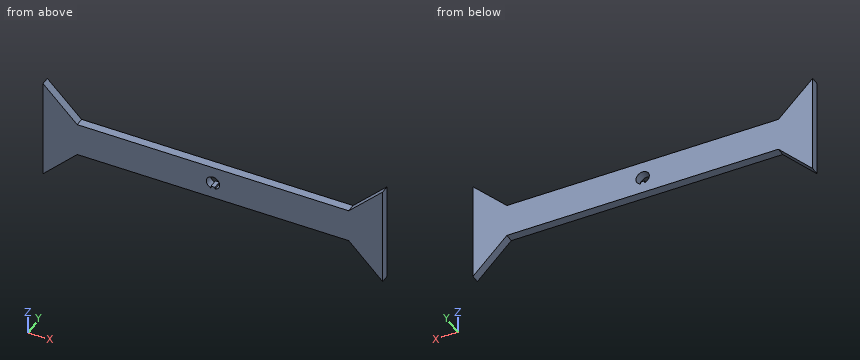
```python
from build123d import *

# Parameters (mm, degrees)
BOSS_EXTRUDE2_DEPTH = 6.35


with BuildPart() as part:
    # Sketch1 → Boss-Extrude2 (new body)
    with BuildSketch(Plane(origin=(0, 0, 0), x_dir=(1, 0, 0), z_dir=(0, 1, 0))):
        Polygon((0, 51.029291752), (0, -25.629291752), (25.629291752, 0), (228.829291752, 0), (254.229291752, -25.094710057), (254.229291752, 51.105289943), (228.829291752, 25.4), (25.629291752, 25.4), align=None)
        with BuildLine():
            Line((125.729291752, 17.77498595), (125.729291752, 16.205289943))
            Line((125.729291752, 16.205289943), (128.729291752, 16.205289943))
            Line((128.729291752, 16.205289943), (128.729291752, 17.77498595))
            ThreePointArc((128.729291752, 17.77498595), (127.229291752, 8.005289943), (125.729291752, 17.77498595))
        make_face(mode=Mode.SUBTRACT)
    extrude(amount=BOSS_EXTRUDE2_DEPTH)


solid = part.part
```
Read the model definition and answer for the solid it produces. Units are mm, in the model's axes. Give positions to 0.01 mm unless a question says otherwise; leave off trailing zeros. Loops run counter-clockwise (first coordinate to the right, second up) from the corner with the lowest first, then second, coordinate; pieces in that order, holes last.
Item 1: The part is cut by section D-D (x = 210). Write down the section's boundary in (y, z), and give its area (3 significant figures).
Item 2: The part is cut by section A-A (y = 2). Write down the section's boundary in (x, z), and give its area (3 significant figures).
Item 3: The part is cut by section C-C (z = 9). Write down the section's boundary in (x, y).
Item 4: Each of these flat-tipped pins is pushed along its axis until it touches: pin 1 Ø1.5 at (x, y) = (211, 1) entering from -Z; pin 2 Ø3.5 at (x, y) = (127, 3) entering from +Z. Where does it stop, or does it pass through?
Item 5: The part is cut by section B-B (z = -12). Write down the section's boundary in (x, y), and give its area (3 significant figures).
Item 6: Find the intervals of material crossed by line 1 along Z through (x, y) = (120, 1.75); line 2 along Z through (x, y) = (131.5, 3.25); line 3 along X through (y, z) = (3, -35), in increasing order.
Taken from the geometry:
1. outline: (0, -25.4) - (6.35, -25.4) - (6.35, 0) - (0, 0) - close
1. area: 161 mm2
2. outline: (0, -51.03) - (25.63, -25.4) - (228.83, -25.4) - (254.23, -51.11) - (254.23, 25.09) - (228.83, 0) - (25.63, 0) - (0, 25.63) - close; hole (125.73, -17.77) - (125.73, -16.21) - (128.73, -16.21) - (128.73, -17.77) arc R5 ccw (long way) to start
2. area: 7,690 mm2
3. outline: (0, 0) - (16.63, 0) - (16.63, 6.35) - (0, 6.35) - close; (237.94, 0) - (254.23, 0) - (254.23, 6.35) - (237.94, 6.35) - close
4. pin 1: stops at z = -25.4
4. pin 2: stops at z = 0
5. outline: (0, 0) - (122.33, 0) - (122.33, 6.35) - (0, 6.35) - close; (132.13, 0) - (254.23, 0) - (254.23, 6.35) - (132.13, 6.35) - close
5. area: 1,550 mm2
6. line 1: z = -25.4 to 0
6. line 2: z = -25.4 to -15.61, -10.41 to 0
6. line 3: x = 0 to 16.03, 238.32 to 254.23
